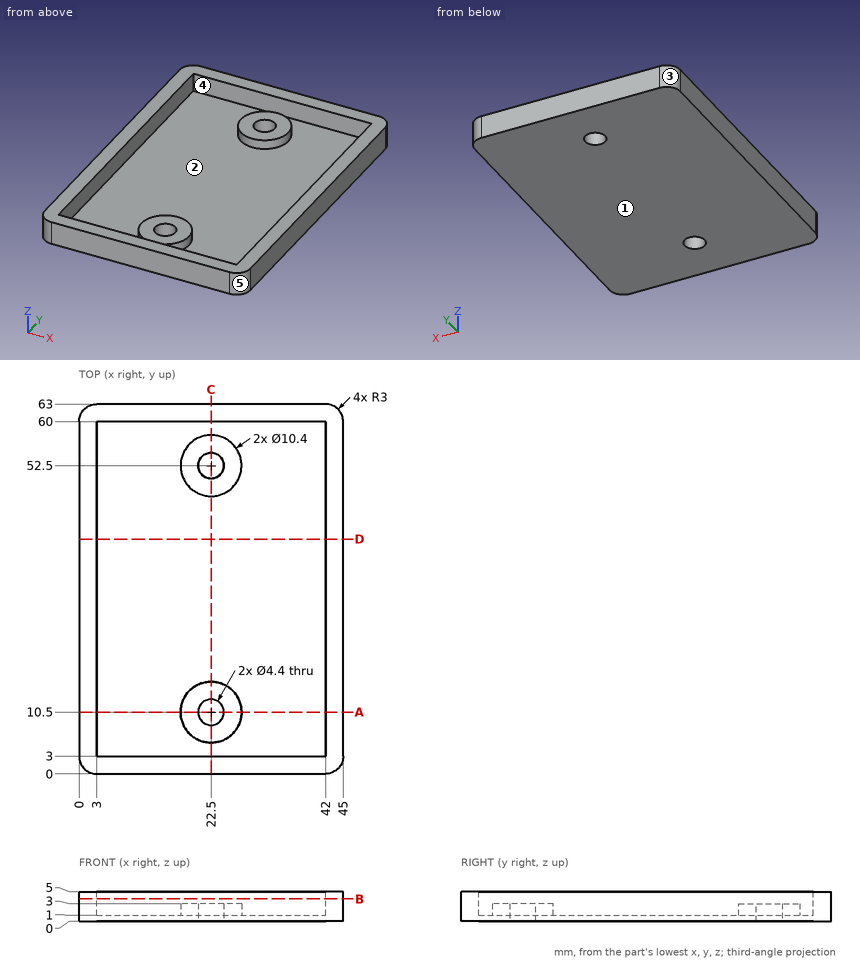
For this review, use the dimensioned drawing (mm, ordinates from the lowest corner) and the shaded views. A direction names the side the tool comes from. Give positions to 0.01 mm unless a question says otherwise; leave off trailing zeros. Write each loop counter-clockwise with the first axis right and the second up, starting at its lowest first coordinate (ties: lowest second). Pieces come first, ordered by that corner, then holes. Notation, with made-up numbers: M 81.25,62 L 122.25,62 A20 ccw 122.25,88 Z; hole C -7,79.25 d7. An arc over 180 degrees is marked long. Answer as a JSON object with one key per item and string values. Group by question number.
Item 1: Draft analysis for pull direction X (two halves, no side actions). For the marked faces 1, 2 and 3, state which applies: +X half, -X half, draft (parallel to the pull), parting line (faces both ways), or undercut.
Item 2: Consider section C-C on x = 22.5. Write out the cut boundary in (y, z).
Item 3: For pin 1 Ø6 at (x, y) = (19, 22) entering from -Z; pin 2 Ø5.5 at (x, y) = (22.5, 10.5) entering from +Z; pin 3 Ø19.5 at (x, y) = (13, 37) entering from +Z, all flat-tipped, find the tip position at first contact; note any pin that passes through.
Item 4: For probe 1 along X at (y, z) = (10.5, 2.2); probe 2 along X at (y, z) = (20, 2.9); probe 3 along Y at (x, z) = (14, 2.95), list the stretches that pass through material, from the lowest coordinate up. Write a range as [from, to].
Item 5: Consider section D-D on y = 40. Write out the cut boundary in (x, z), plus the area to 3 significant figures.
Item 6: Consider section B-B on z = 3.8. Write out the cut boundary in (x, y).
Item 7: Consider section A-A on y = 10.5. Write out the cut boundary in (x, z).
Item 8: Tool access review of the marked faces 4 and 5: name each direction out of +Z, -Z, +X, -X, +Y, -Y from which nothing blocks a thin tool from reaching the whole face with its end or side.
Check result:
{
 "1": {"face 1": "draft", "face 2": "undercut", "face 3": "-X half"},
 "2": {"outline": "M 0,0 L 8.3,0 L 8.3,3 L 5.3,3 L 5.3,1 L 3,1 L 3,5 L 0,5 Z; M 12.7,0 L 50.3,0 L 50.3,3 L 47.3,3 L 47.3,1 L 15.7,1 L 15.7,3 L 12.7,3 Z; M 54.7,0 L 63,0 L 63,5 L 60,5 L 60,1 L 57.7,1 L 57.7,3 L 54.7,3 Z"},
 "3": {"pin 1": "stops at z = 0", "pin 2": "stops at z = 3", "pin 3": "stops at z = 1"},
 "4": {"probe 1": "x = [0, 3], [17.3, 20.3], [24.7, 27.7], [42, 45]", "probe 2": "x = [0, 3], [42, 45]", "probe 3": "y = [0, 3], [60, 63]"},
 "5": {"outline": "M 0,0 L 45,0 L 45,5 L 42,5 L 42,1 L 3,1 L 3,5 L 0,5 Z", "area": "69.0 mm^2"},
 "6": {"outline": "M 0,3 A3 ccw 3,0 L 42,0 A3 ccw 45,3 L 45,60 A3 ccw 42,63 L 3,63 A3 ccw 0,60 Z; hole M 3,3 L 42,3 L 42,60 L 3,60 Z"},
 "7": {"outline": "M 0,0 L 20.3,0 L 20.3,3 L 17.3,3 L 17.3,1 L 3,1 L 3,5 L 0,5 Z; M 24.7,0 L 45,0 L 45,5 L 42,5 L 42,1 L 27.7,1 L 27.7,3 L 24.7,3 Z"},
 "8": {"face 4": "+Z", "face 5": "+Z, -Z, +X, -Y"}
}
